Here's how the part is built. I have some questions about the finished solid (model axes, mm). A direction names the side the tool comes from. Give positions to 0.01 mm unless a question says otherwise; leave off trailing zeros. Loops run counter-clockwise (first coordinate to the right, second up) from the corner with the lowest first, then second, coordinate; pieces in that order, holes last. Notation, with made-up numbers: (53.25, 51) - (76.25, 51) arc R6 ccw to (76.25, 61) - close; hole circle Ø10 at (-23, 59). An arc over 180 degrees is marked (long way). Return JSON: item names as keys, results as strings. Group by question number.
(1) On a 3-axis mill with a long thin cutter (end or side, diameter ignored), from which of +Z, -Z, +X, -X, +Y, -Y can I reach the whole of each face in a straight line? I mean faces 4 (the cylindrical face through (19.479, 14.466, -9.86)), 5 (the flat face through (37.2, 3, -10.1)), 6 (the flat face through (7.2, 3, -10.1)). Say none if no direction works.
(2) I need wall thicknesses on probe 1 along X at (y, z) = (1.35, -10); probe 2 along Y at (x, z) = (20, -14.5); probe 3 along X at (y, z) = (12, -15). Which ranges of each line are inside material? Lowest first, please. Write a range as [from, to].
(3) If we section it at A-A (z = -10): State how many separate pieces and enclosed holes the cut face has, then the cut area to 3 significant figures.
(4) If we mould it in two halves opening along X, with no side actions, what happens to faces 1 (the cylindrical face through (5, 2, -12)), 2 (the flat face through (20, 0, -10)), 3 (the flat face through (0, 1, -10))? For each: released by +X, released by -X, zero draft, split by the parting line, or undercut.
(5) If we section it at B-B (x = 5): Please give me the cut outline in (y, z).
(6) For P1, Ø1.5, axis at y = 5, z = -6.5, coming from the -X side; P2, Ø2, axis at x = 12, z = -10.5, coming from the +Y side; P3, Ø6.5, axis at x = 35, z = -10, coming from the +Y side; P4, Ø10, axis at y = 3.5, z = -16, coming from the +X side, each with a flat end and sliding along its axis, tell me the tip position at first contact or that it passes through.
(7) If we section it at C-C (y = 1.75): Please give me the cut outline in (x, z), then the cut area to 3 significant figures.
(8) If we section it at D-D (y = 8.75): Please give me the cut outline in (x, z), then the cut area to 3 significant figures.
```python
from build123d import *

# Parameters (mm, degrees)
SKETCH1_W           = 40
SKETCH1_H           = 20
BOSS_EXTRUDE1_DEPTH = 3
SKETCH2_W           = 20
SKETCH2_H           = 20
BOSS_EXTRUDE2_DEPTH = 15
SKETCH3_R           = 4
CUT_EXTRUDE1_DEPTH  = 49.207883173
FILLET1_R           = 10
SKETCH4_R           = 2
CUT_EXTRUDE2_DEPTH  = 48.16990566


with BuildPart() as part:
    # Sketch1 → Boss-Extrude1 (new body)
    with BuildSketch(Plane(origin=(0, 0, 0), x_dir=(1, 0, 0), z_dir=(0, 1, 0))):
        with Locations((20, 10)):
            Rectangle(SKETCH1_W, SKETCH1_H)
    extrude(amount=BOSS_EXTRUDE1_DEPTH)

    # Sketch2 → Boss-Extrude2 (add)
    with BuildSketch(Plane(origin=(0, 3, 0), x_dir=(1, 0, 0), z_dir=(0, 1, 0))):
        with Locations((20, 10)):
            Rectangle(SKETCH2_W, SKETCH2_H)
    extrude(amount=BOSS_EXTRUDE2_DEPTH)

    # Sketch3 → Cut-Extrude1 (cut, through all)
    with BuildSketch(Plane.XY):
        with Locations((20, 10.5)):
            Circle(SKETCH3_R)
    extrude(amount=-CUT_EXTRUDE1_DEPTH, mode=Mode.SUBTRACT)

    # Fillet1
    fillet1_edges = [part.edges().sort_by_distance(p)[0] for p in [
        (30, 18, -10),
        (10, 18, -10),
    ]]
    fillet(fillet1_edges, radius=FILLET1_R - 0.0001)  # a hair under: the kernel refuses the full size

    # Sketch4 → Cut-Extrude2 (cut, through all)
    with BuildSketch(Plane(origin=(0, 3, 0), x_dir=(1, 0, 0), z_dir=(0, 1, 0))):
        with Locations(Location((35, 10, 0), (0, 0, 270))):
            Circle(SKETCH4_R)
        with Locations(Location((5, 10, 0), (0, 0, 270))):
            Circle(SKETCH4_R)
    extrude(amount=-CUT_EXTRUDE2_DEPTH, mode=Mode.SUBTRACT)


solid = part.part
```
Values:
{
 "1": {"face 4": "+Z, -Z", "face 5": "+Z, -Z, +X, +Y", "face 6": "+Z, -Z, -X, +Y"},
 "2": {"probe 1": "[0, 3], [7, 33], [37, 40]", "probe 2": "[0, 6.5], [14.5, 18]", "probe 3": "[10.83, 16.29], [23.71, 29.17]"},
 "3": {"separate pieces": "3", "enclosed holes": "1", "area": "303 mm2"},
 "4": {"face 1": "undercut", "face 2": "zero draft", "face 3": "released by -X"},
 "5": {"outline": "(0, -20) - (3, -20) - (3, -12) - (0, -12) - close; (0, -8) - (3, -8) - (3, 0) - (0, 0) - close"},
 "6": {"P1": "x = 10", "P2": "y = 15.14", "P3": "y = 3", "P4": "x = 40"},
 "7": {"outline": "(0, -20) - (40, -20) - (40, 0) - (0, 0) - close; hole circle Ø4 at (5, -10); hole circle Ø4 at (35, -10)", "area": "775 mm2"},
 "8": {"outline": "(10.03, -20) - (16.4, -20) - (16.4, 0) - (10.03, 0) - close; (23.6, -20) - (29.97, -20) - (29.97, 0) - (23.6, 0) - close", "area": "255 mm2"}
}
